from build123d import *

# Parameters (mm, degrees)
BOSS_EXTRUDE1_DEPTH = 20
CHAMFER1_SIZE       = 10
FILLET1_R           = 10
FILLET2_R           = 10
SKETCH9_W           = 105
SKETCH9_H           = 30
CUT_EXTRUDE2_DEPTH  = 109.656569187


with BuildPart() as part:
    # Sketch1 → Boss-Extrude1 (new body)
    with BuildSketch(Plane.XY):
        with BuildLine():
            Line((-37.5, 0), (-37.5, -100))
            Line((-37.5, -100), (37.5, -100))
            Line((37.5, -100), (37.5, 0))
            ThreePointArc((37.5, 0), (0, 37.5), (-37.5, 0))
        make_face()
    extrude(amount=BOSS_EXTRUDE1_DEPTH)

    # Chamfer1
    chamfer1_edges = [part.edges().sort_by_distance(p)[0] for p in [
        (-37.5, -50, 20),
        (0, 37.5, 20),
        (37.5, -50, 20),
    ]]
    chamfer(chamfer1_edges, length=CHAMFER1_SIZE)

    # Fillet1
    fillet1_edges = [part.edges().sort_by_distance(p)[0] for p in [
        (-27.5, -50, 20),
        (0, 27.5, 20),
        (27.5, -50, 20),
    ]]
    fillet(fillet1_edges, radius=FILLET1_R)

    # Fillet2
    fillet2_edges = [part.edges().sort_by_distance(p)[0] for p in [
        (37.5, -50, 10),
        (0, 37.5, 10),
        (-37.5, -50, 10),
    ]]
    fillet(fillet2_edges, radius=FILLET2_R)

    # Sketch9 → Cut-Extrude2 (cut, through all)
    with BuildSketch(Plane(origin=(0, 0, 0), x_dir=(-1, 0, 0), z_dir=(0, 0, -1))):
        with Locations((0, -90)):
            Rectangle(SKETCH9_W, SKETCH9_H)
    extrude(amount=-CUT_EXTRUDE2_DEPTH, mode=Mode.SUBTRACT)


solid = part.part
Design review of the part built by this model. Coordinates are the model's own, in mm. Coordinates: 2 decimals unless noted, no trailing zeros. Loops run counter-clockwise (first coordinate to the right, second up) from the corner with the lowest first, then second, coordinate; pieces in that order, holes last. Notation, with made-up numbers: M 39.5,55.25 L 49.5,55.25 A29 ccw 49.5,78.25 Z; hole C -8.75,32 d11. An arc over 180 degrees is marked long. Answer as CSV lines item,"result".
Item 1: Add section C-C on z = 18.75. State the section outline as (x, y) points.
Answer list:
outline,"M -28.2,-75 L 28.2,-75 L 28.2,0 A28.2 ccw -28.2,0 Z"
Item 2: For P1, Ø2, axis at y = -36, z = 11, coming from the -X side; P2, Ø3, axis at y = 15.5, z = 16.5, coming from the +X side, all flat-tipped, find the tip position at first contact; note any pin that passes through.
Answer list:
P1,"x = -36.6"
P2,"x = 28.74"
Item 3: Add section B-B on z = 4.25. State the section outline as (x, y) points.
Answer list:
outline,"M -37.5,-75 L 37.5,-75 L 37.5,0 A37.5 ccw -37.5,0 Z"
Item 4: For probe 1 along Z at (x, y) = (-23.5, -1); probe 2 along X at (y, z) = (-61, 8.25); probe 3 along X at (y, z) = (24.5, 18), list the stretches that pass through material, from the lowest coordinate up.
Answer list:
probe 1,"0 to 20"
probe 2,"-37.21 to 37.21"
probe 3,"-16.18 to 16.18"
Item 5: Add section A-A on y = -49.5. State the section outline as (x, z) points.
Answer list:
outline,"M -37.5,0 L 37.5,0 L 37.5,5.86 A10 ccw 34.57,12.93 L 30.43,17.07 A10 ccw 23.36,20 L -23.36,20 A10 ccw -30.43,17.07 L -34.57,12.93 A10 ccw -37.5,5.86 Z"
